```python
from build123d import *

# Parameters (mm, degrees)
Y_KSEKLIK_EKSTR_ZYON2_DEPTH       = 14
KES_EKSTR_ZYON1_REACH             = 39.5
IZIM2_R                           = 2.75
KES_EKSTR_ZYON1_DIRECTION_2_DEPTH = 1


with BuildPart() as part:
    # Çizim1 → Yükseklik-Ekstrüzyon2 (new body)
    with BuildSketch(Plane.XY):
        with BuildLine():
            Line((21, -23), (-21, -23))
            Line((-21, -23), (-21, -16.5))
            Line((-21, -16.5), (-10, -16.5))
            Line((-10, -16.5), (-10, 14.5))
            Line((-10, 14.5), (-0.5, 14.5))
            Line((-0.5, 14.5), (-0.5, 5.979130372))
            ThreePointArc((-0.5, 5.979130372), (0, -6), (0.5, 5.979130372))
            Line((0.5, 5.979130372), (0.5, 14.5))
            Line((0.5, 14.5), (10, 14.5))
            Line((10, 14.5), (10, -16.5))
            Line((10, -16.5), (21, -16.5))
            Line((21, -16.5), (21, -23))
        make_face()
    extrude(amount=Y_KSEKLIK_EKSTR_ZYON2_DEPTH)

    # Çizim2 → Kes-Ekstrüzyon1 (cut, up to next)
    with BuildSketch(Plane.XZ.offset(23), mode=Mode.PRIVATE) as kes_ekstr_zyon1_sk1:
        with Locations((-16, 7)):
            Circle(IZIM2_R)
    kes_ekstr_zyon1_tool1 = extrude(kes_ekstr_zyon1_sk1.sketch, amount=-KES_EKSTR_ZYON1_REACH, mode=Mode.PRIVATE) & part.part
    add(kes_ekstr_zyon1_tool1.solids().sort_by_distance((-16, -23, 7))[0], mode=Mode.SUBTRACT)
    # Çizim2 → Kes-Ekstrüzyon1 (cut, up to next)
    with BuildSketch(Plane.XZ.offset(23), mode=Mode.PRIVATE) as kes_ekstr_zyon1_sk2:
        with Locations((16, 7)):
            Circle(IZIM2_R)
    kes_ekstr_zyon1_tool2 = extrude(kes_ekstr_zyon1_sk2.sketch, amount=-KES_EKSTR_ZYON1_REACH, mode=Mode.PRIVATE) & part.part
    add(kes_ekstr_zyon1_tool2.solids().sort_by_distance((16, -23, 7))[0], mode=Mode.SUBTRACT)

    # Çizim2 → Kes-Ekstrüzyon1 direction 2 (cut)
    with BuildSketch(Plane.XZ.offset(23)):
        with Locations((-16, 7)):
            Circle(IZIM2_R)
        with Locations((16, 7)):
            Circle(IZIM2_R)
    extrude(amount=KES_EKSTR_ZYON1_DIRECTION_2_DEPTH, mode=Mode.SUBTRACT)


solid = part.part
```
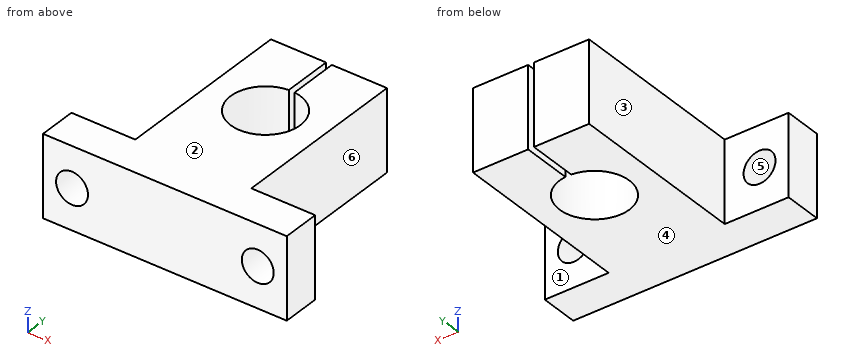
Could you check a few things on this model? Use its own coordinates, in mm. Face numbers are marked on the shaded views. A direction names the side the tool comes from. Give positions to 0.01 mm unless a question says otherwise; leave off trailing zeros. Order: outer loops, then holes, each group sorted by start corner. A loop starts at its lowest first (then second) coordinate and runs counter-clockwise, first axis right, second up.
Q1. Suppose I cut it at A-A, the plane y = 0. Write out the boundary of the cut face in (x, z), and give its area (3 significant figures).
Q2. For the marked faces 1, 2 and 3, which set-ups out of +Z, -Z, +X, -X, +Y, -Y let a thin tool reach every point of the face, with its end or its side?
Q3. I'm going to push flat-ended pins straight in: P1, Ø1, axis at y = -7.5, z = 3, coming from the +X side; P2, Ø5.5, axis at x = -14.5, z = 7, coming from the +Y side; P3, Ø1, axis at y = -6.5, z = 4.5, coming from the -X side; P4, Ø7, axis at x = 0, y = 0, coming from the +Z side. Where does each tip first touch, or does it pass through?
Q4. Suppose I cut it at C-C, the plane z = 7. Write out the boundary of the cut face in (x, y).
Q5. Suppose I cut it at D-D, the plane y = -19. Write out the boundary of the cut face in (x, z), and give its area (3 significant figures).
Q6. We'd pull the mould along Z, two halves only. Please class the marked faces 4, 5 and 6: +Z half, -Z half, draft (parallel to the pull), parting line (faces both ways), or undercut.
Q7. Suppose I cut it at B-B, the plane x = -16. Write out the boundary of the cut face in (y, z).
Q8. If I drill on line 1 along X through (y, z) = (0, 4); line 2 along X through (y, z) = (11, 2.5); line 3 along Z through (x, y) = (16, -19), over which ranges is the centre line in solid material (lowest first)?
Solution:
1. outline: (-10, 0) - (-6, 0) - (-6, 14) - (-10, 14) - close; (6, 0) - (10, 0) - (10, 14) - (6, 14) - close
1. area: 112 mm2
2. face 1: +Z, -Z, +X, +Y
2. face 2: +Z, +X, -X, +Y, -Y
2. face 3: +Z, -Z, -X, +Y
3. P1: stops at x = 10
3. P2: stops at y = -16.5
3. P3: stops at x = -10
3. P4: passes through
4. outline: (-21, -23) - (-18.75, -23) - (-18.75, -16.5) - (-21, -16.5) - close; (-13.25, -23) - (13.25, -23) - (13.25, -16.5) - (10, -16.5) - (10, 14.5) - (0.5, 14.5) - (0.5, 5.98) arc R6 cw (long way) to (-0.5, 5.98) - (-0.5, 14.5) - (-10, 14.5) - (-10, -16.5) - (-13.25, -16.5) - close; (18.75, -23) - (21, -23) - (21, -16.5) - (18.75, -16.5) - close
5. outline: (-21, 0) - (21, 0) - (21, 14) - (-21, 14) - close; hole circle Ø5.5 at (-16, 7); hole circle Ø5.5 at (16, 7)
5. area: 540 mm2
6. face 4: -Z half
6. face 5: undercut
6. face 6: draft
7. outline: (-23, 0) - (-16.5, 0) - (-16.5, 4.25) - (-23, 4.25) - close; (-23, 9.75) - (-16.5, 9.75) - (-16.5, 14) - (-23, 14) - close
8. line 1: x = -10 to -6, 6 to 10
8. line 2: x = -10 to -0.5, 0.5 to 10
8. line 3: z = 0 to 4.25, 9.75 to 14
